Source: CAD feature listing. Evaluate the final solid. Frame: model axes, mm. Give positions to 0.01 mm unless a question says otherwise; leave off trailing zeros. Order: outer loops, then holes, each group sorted by start corner. A loop starts at its lowest first (then second) coordinate and runs counter-clockwise, first axis right, second up. Notation, with made-up numbers: (28, 76) -> (61, 76) arc R28 cw to (61, 108) -> close; hole circle Ø10 at (51, -33). An arc over 180 degrees is marked (long way). Use CSV: the item, a comma, the result in double quotes.
Autodesk Inventor part; units mm, degrees
ref_plane "YZ Plane" through (0, 0, 0) normal (1, 0, 0) x (0, 1, 0)
ref_plane "XZ Plane" through (0, 0, 0) normal (0, 1, 0) x (-1, 0, 0)
ref_plane "XY Plane" through (0, 0, 0) normal (0, 0, 1) x (1, 0, 0)
ref_plane "작업 평면2" through (-1.8693, 3.0801, 0) normal (0, 0, 1) x (0.9953009, -0.0968305, 0)
sketch "스케치1" plane through (-1.8693, 3.0801, 0) normal (0, 0, 1) x (0.9953009, -0.0968305, 0)
  line L0 (44.1285, 26.3164) -> (48.97, -23.4487)
  line L1 (49.551, -29.4205) -> (48.97, -23.4487)
  line L2 (55.5228, -28.8395) -> (-45.2017, -38.6387)
  line L3 (49.5193, 32.8692) -> (55.5228, -28.8395)
  line L4 (-51.2052, 23.0699) -> (49.5193, 32.8692)
  line L5 (44.1285, 26.3164) -> (43.5475, 32.2882)
  point P0 (2.1588, -2.8846)
extrude "돌출1" add sketch "스케치1" along normal blind 35
sketch "스케치2" plane through (-1.8693, 3.0801, 0) normal (0, 0, -1) x (-0.9953009, 0.0968305, 0)
  circle A0 centre (-48.7397, 9.9006) radius 1.35
  circle A1 centre (-50.8699, -11.996) radius 1.35
  point P0 (-2.1588, -2.8846)
extrude "돌출2" cut sketch "스케치2" against normal blind 5
ref_plane "작업 평면3" through (50.6, -31.0001, 0) normal (1, 0, 0) x (0, 0, -1)
sketch "스케치3" plane through (50.6, -31.0001, 0) normal (1, 0, 0) x (0, 0, -1)
  line L0 (-5, 40.5649) -> (-5, 37.8649)
  line L1 (-5, 18.5649) -> (-5, 15.8649)
  line L2 (-4, 0) -> (-4, 6)
  line L3 (-4, 1.65) -> (0, 1.65)
  line L4 (-4, 4.35) -> (0, 4.35)
  line L5 (-4, 37.2149) -> (-4, 41.2149)
  line L6 (-4, 41.2149) -> (-6, 41.2149)
  line L7 (-6, 41.2149) -> (-6, 37.2149)
  line L8 (-6, 37.2149) -> (-4, 37.2149)
  line L9 (-4, 37.2149) -> (-6, 41.2149) construction
  line L10 (-4, 41.2149) -> (-6, 37.2149) construction
  line L11 (-4, 15.2149) -> (-4, 19.2149)
  line L12 (-4, 19.2149) -> (-6, 19.2149)
  line L13 (-6, 19.2149) -> (-6, 15.2149)
  line L14 (-6, 15.2149) -> (-4, 15.2149)
  line L15 (-4, 15.2149) -> (-6, 19.2149) construction
  line L16 (-4, 19.2149) -> (-6, 15.2149) construction
  point P0 (0, 31.0001)
  point P1 (-5, 39.2149)
  point P2 (-5, 17.2149)
  dimension "d4" = 4
  dimension "d5" = 2
  dimension "d6" = 4
extrude "돌출3" cut sketch "스케치3" against normal up to surface (6 mm away)
properties part number "_head_adt_2" material "PMMA 플라스틱"
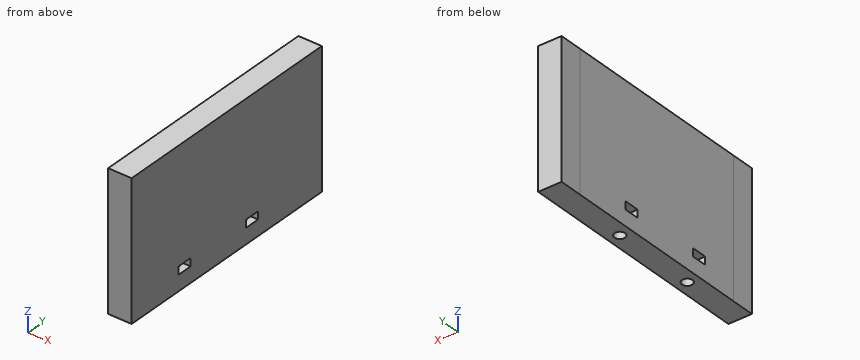
1. Section query B-B on x = 47.25. Return loops of the section in (y, z), plus the area to 3 significant figures.
Answer below:
outline,"(-31, 0) -> (-15.09, 0) -> (-15.09, 4) -> (-15.79, 4) -> (-15.79, 6) -> (-11.79, 6) -> (-11.79, 4) -> (-12.48, 4) -> (-12.48, 0) -> (6.91, 0) -> (6.91, 4) -> (6.21, 4) -> (6.21, 6) -> (10.21, 6) -> (10.21, 4) -> (9.52, 4) -> (9.52, 0) -> (31, 0) -> (31, 35) -> (-31, 35) -> close"
area,"2,130 mm²"
2. Section query A-A on z = 2. Return loops of the section in (x, y).
Answer below:
outline,"(44.6, -31) -> (50.6, -31) -> (50.6, 31) -> (44.6, 31) -> (44.6, 25) -> (44.6, -25) -> close; hole circle Ø2.7 at (47.6, -13.79); hole circle Ø2.7 at (47.6, 8.21)"
3. Ray query, line 1 along Y through (x, z) = (47.5, 5.5); line 2 along Y through (x, z) = (48, 2); line 3 along Z through (x, y) = (49.5, 9). Return the intervals inside material, ascending.
Answer below:
line 1,"y = -31 to -15.79, -11.79 to 6.21, 10.21 to 31"
line 2,"y = -31 to -15.07, -12.5 to 6.93, 9.5 to 31"
line 3,"z = 0 to 4, 6 to 35"
